The listing builds one solid part. Answer for the finished solid, in the listing's coordinates (mm). Round coordinates to 2 decimals unless told otherwise and drop trailing zeros. Order: outer loops, then holes, each group sorted by start corner. A loop starts at its lowest first (then second) coordinate and runs counter-clockwise, first axis right, second up. Notation, with made-up numbers: (84.25, -9) -> (120.25, -9) arc R17 ccw to (120.25, 8) -> close; hole circle Ø1 at (21.5, 18.5). An arc over 180 degrees is marked (long way). Answer in a Markdown table with one row per item. Add a question column.
```python
from build123d import *

# Parameters (mm, degrees)
ESQUISSE2_R        = 1.5
ESQUISSE2_R_2      = 2.5
BOSS_EXTRU_1_DEPTH = 5


with BuildPart() as part:
    # Esquisse2 → Boss.-Extru.1 (new body)
    with BuildSketch(Plane.XZ.offset(38.8)):
        with BuildLine():
            Line((8.857142857, -0.065520771), (-25.685714286, -4.039312463))
            ThreePointArc((-25.685714286, -4.039312463), (-31, -10), (-25.685714286, -15.960687537))
            Line((-25.685714286, -15.960687537), (8.857142857, -19.934479229))
            Line((8.857142857, -19.934479229), (30.467410963, -24.355663986))
            ThreePointArc((30.467410963, -24.355663986), (32.607632, 0.67215889), (11.924183808, 14.92584034))
            Line((11.924183808, 14.92584034), (8.857142857, -0.065520771))
        make_face()
        with Locations(Location((10, -10, 0), (0, 0, 270))):
            Circle(ESQUISSE2_R, mode=Mode.SUBTRACT)
        with Locations(Location((-25, -10, 0), (0, 0, 270))):
            Circle(ESQUISSE2_R_2, mode=Mode.SUBTRACT)
    extrude(amount=BOSS_EXTRU_1_DEPTH)


solid = part.part
```
Item 1: The part is cut by section D-D, the plane x = -25. Give the vertices of the cut face in (y, z).
Item 2: The part is cut by section A-A, the plane z = -10. Give the vertices of the cut face in (x, y).
Item 3: Find the intervals of material crossed by probe 1 along X at (y, z) = (-40.1, -11); probe 2 along X at (y, z) = (-40.5, -9.5) (3 decimals); probe 3 along X at (y, z) = (-40.85, -8), in increasing order. Write a range as [from, to].
Item 4: The part is cut by section B-B, the plane x = 10. Give the vertices of the cut face in (y, z), and give its area (3 significant figures).
Item 5: The part is cut by section C-C, the plane y = -40.9. Give the vertices of the cut face in (x, z).
Item 6: Flat-ended cylindrical pins translate along their axes: P1, Ø1.5, axis at x = -10, y = -40, coming from the +Z side; P2, Ø1, axis at y = -39.5, z = -13.5, coming from the +X side; P3, Ø1, axis at x = -17.5, y = -40.5, coming from the +Z side. Find the tip coordinate at first contact, or state that the pin passes through.
Item 7: For a pull along Z with two mould halves and no side action, classify faces 1 (the face through (32.76, -41.26, 0.34)), 2 (the face through (-22.52, -41.26, -9.67)), 3 (the face through (19.511, -41.265, -22.114)), 4 (the face through (9, -38.8, -4)) as released by +Z, released by -Z, zero draft, split by the parting line, or undercut.
Resolved:
| question | item | result |
|---|---|---|
| 1 | outline | (-43.8, -16.04) -> (-38.8, -16.04) -> (-38.8, -12.5) -> (-43.8, -12.5) -> close; (-43.8, -7.5) -> (-38.8, -7.5) -> (-38.8, -3.96) -> (-43.8, -3.96) -> close |
| 2 | outline | (-31, -43.8) -> (-27.5, -43.8) -> (-27.5, -38.8) -> (-31, -38.8) -> close; (-22.5, -43.8) -> (8.5, -43.8) -> (8.5, -38.8) -> (-22.5, -38.8) -> close; (11.5, -43.8) -> (35, -43.8) -> (35, -38.8) -> (11.5, -38.8) -> close |
| 3 | probe 1 | [-30.92, -27.29], [-22.71, 8.88], [11.12, 34.98] |
| 3 | probe 2 | [-30.979, -27.449], [-22.551, 8.586], [11.414, 34.995] |
| 3 | probe 3 | [-30.66, -26.5], [-23.5, 34.92] |
| 4 | outline | (-43.8, -20.17) -> (-38.8, -20.17) -> (-38.8, -11.5) -> (-43.8, -11.5) -> close; (-43.8, -8.5) -> (-38.8, -8.5) -> (-38.8, 5.52) -> (-43.8, 5.52) -> close |
| 4 | area | 113 mm2 |
| 5 | outline | (-25.69, -15.96) -> (8.86, -19.93) -> (30.47, -24.36) arc R25 ccw to (11.92, 14.93) -> (8.86, -0.07) -> (-25.69, -4.04) arc R6 ccw to start; hole circle Ø5 at (-25, -10); hole circle Ø3 at (10, -10) |
| 6 | P1 | z = -2.15 |
| 6 | P2 | x = 34.82 |
| 6 | P3 | z = -3.04 |
| 7 | face 1 | split by the parting line |
| 7 | face 2 | undercut |
| 7 | face 3 | released by -Z |
| 7 | face 4 | zero draft |
